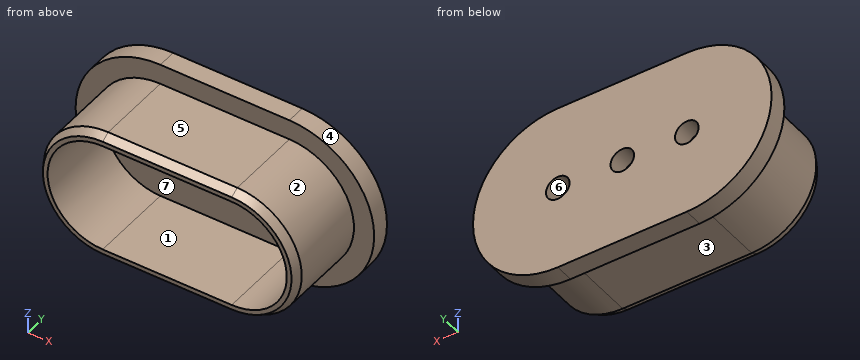
from build123d import *

# Parameters (mm, degrees)
BOSS_EXTRUDE1_DEPTH     = 4.5
SKETCH2_R               = 0.625
BOSS_EXTRUDE2_DEPTH     = 1
CHAMFER2_SIZE           = 0.25
CHAMFER2_SIZE2          = 0.433012702
SKETCH3_R               = 0.625
CUT_EXTRUDE1_DEPTH      = 1
CUT_EXTRUDE1_DEPTH_BACK = 6.5


with BuildPart() as part:
    # Sketch1 → Boss-Extrude1 (new body)
    with BuildSketch(Plane(origin=(0, 0, 0), x_dir=(1, 0, 0), z_dir=(0, 1, 0))):
        with BuildLine():
            Line((-3.425, 3.425), (3.425, 3.425))
            ThreePointArc((3.425, 3.425), (6.85, 0), (3.425, -3.425))
            Line((3.425, -3.425), (-3.425, -3.425))
            ThreePointArc((-3.425, -3.425), (-6.85, 0), (-3.425, 3.425))
        make_face()
        with BuildLine():
            Line((-3.425, 2.925), (3.425, 2.925))
            ThreePointArc((3.425, 2.925), (6.35, 0), (3.425, -2.925))
            Line((3.425, -2.925), (-3.425, -2.925))
            ThreePointArc((-3.425, -2.925), (-6.35, 0), (-3.425, 2.925))
        make_face(mode=Mode.SUBTRACT)
    extrude(amount=BOSS_EXTRUDE1_DEPTH)

    # Sketch2 → Boss-Extrude2 (add)
    with BuildSketch(Plane(origin=(0, 4.5, 0), x_dir=(1, 0, 0), z_dir=(0, 1, 0))):
        with BuildLine():
            Line((-3.425, 4.5), (3.425, 4.5))
            ThreePointArc((3.425, 4.5), (7.925, 0), (3.425, -4.5))
            Line((3.425, -4.5), (-3.425, -4.5))
            ThreePointArc((-3.425, -4.5), (-7.925, 0), (-3.425, 4.5))
        make_face()
        with Locations((-3.425, 0)):
            Circle(SKETCH2_R, mode=Mode.SUBTRACT)
        with Locations((3.425, 0)):
            Circle(SKETCH2_R, mode=Mode.SUBTRACT)
    extrude(amount=BOSS_EXTRUDE2_DEPTH)

    # Chamfer2
    chamfer2_edges = [part.edges().sort_by_distance(p)[0] for p in [
        (0, 0, 3.425),
        (-6.85, 0, 0),
        (0, 0, -3.425),
        (6.85, 0, 0),
    ]]
    chamfer2_side = [part.faces().sort_by_distance(p)[0] for p in [
        (0, 0, -3.271829344),
    ]]
    chamfer(chamfer2_edges, length=CHAMFER2_SIZE, length2=CHAMFER2_SIZE2, reference=chamfer2_side[0])

    # Sketch3 → Cut-Extrude1 (cut, two sides)
    with BuildSketch(Plane(origin=(0, 5.5, 0), x_dir=(1, 0, 0), z_dir=(0, 1, 0))) as cut_extrude1_sk:
        Circle(SKETCH3_R)
    extrude(amount=CUT_EXTRUDE1_DEPTH, mode=Mode.SUBTRACT)
    extrude(cut_extrude1_sk.sketch, amount=-CUT_EXTRUDE1_DEPTH_BACK, mode=Mode.SUBTRACT)


solid = part.part
Model file for the job. Use its own axes, mm. Face numbers are marked on the shaded views. A direction names the side the tool comes from. Give positions to 0.01 mm unless a question says otherwise; leave off trailing zeros. Write each loop counter-clockwise with the first axis right and the second up, starting at its lowest first coordinate (ties: lowest second). Pieces come first, ordered by that corner, then holes. Notation, with made-up numbers: (88.25, 87) -> (124.25, 87) arc R21 cw to (124.25, 108) -> close; hole circle Ø10 at (42.5, 48). An arc over 180 degrees is marked (long way). Write item = value, one per line.
(1) Slice it at A-A, the plane x = 0. Give the cut face in (y, z) (3 decimals).
Determined:
outline = (0, -3.175) -> (0.433, -3.425) -> (4.5, -3.425) -> (4.5, -4.5) -> (5.5, -4.5) -> (5.5, -0.625) -> (4.5, -0.625) -> (4.5, -2.925) -> (0, -2.925) -> close; (0, 2.925) -> (4.5, 2.925) -> (4.5, 0.625) -> (5.5, 0.625) -> (5.5, 4.5) -> (4.5, 4.5) -> (4.5, 3.425) -> (0.433, 3.425) -> (0, 3.175) -> close
(2) Mould opens along Z. For the marked faces 4, 5, 6 and 7 say: released by +Z, released by -Z, zero draft, split by the parting line, or undercut.
Determined:
face_4 = split by the parting line
face_5 = released by +Z
face_6 = undercut
face_7 = undercut
(3) Tool access for the marked faces 1, 2 and 3: list every direction of +Z, -Z, +X, -X, +Y, -Y with a clear straight run to the whole face (end or side of a thin tool).
Determined:
face_1 = -Y
face_2 = +X, -Y
face_3 = -Z, +X, -X, -Y
(4) Probe line 1 along X through (y, z) = (4.9, 0) (3 decimals); line 2 along Z through (x, y) = (-3.5, 3.9); line 3 along Z through (x, y) = (0, 5.25) (3 decimals). List the from-to ranges inside material, lowest first.
Determined:
line_1 = -7.925 to -4.05, -2.8 to -0.625, 0.625 to 2.8, 4.05 to 7.925
line_2 = -3.42 to -2.92, 2.92 to 3.42
line_3 = -4.5 to -0.625, 0.625 to 4.5
(5) Slice it at D-D, the plane y = 4.9. Give the cut face in (x, z) (3 decimals).
Determined:
outline = (-3.425, -4.5) -> (3.425, -4.5) arc R4.5 ccw to (3.425, 4.5) -> (-3.425, 4.5) arc R4.5 ccw to start; hole circle Ø1.25 at (-3.425, 0); hole circle Ø1.25 at (0, 0); hole circle Ø1.25 at (3.425, 0)
(6) Flat gauge pins, fed straight in: P1, Ø1.2, axis at x = 0, y = 2, coming from the -Z side (3 decimals); P2, Ø1.5, axis at x = 5, z = -1, coming from the -Y side; P3, Ø2, axis at x = 3.425, z = 0, coming from the +Y side; P4, Ø3, axis at y = 4.5, z = 2.5, coming from the +X side. Where does each tip first touch, or does it go through?
Determined:
P1 = -3.425
P2 = 4.5
P3 = 5.5
P4 = 7.81
(7) Slice it at C-C, the plane y = 3.35. Give the cut face in (x, z) (3 decimals), then the cut area to 3 significant figures.
Determined:
outline = (-3.425, -3.425) -> (3.425, -3.425) arc R3.425 ccw to (3.425, 3.425) -> (-3.425, 3.425) arc R3.425 ccw to start; hole (-3.425, -2.925) -> (3.425, -2.925) arc R2.925 ccw to (3.425, 2.925) -> (-3.425, 2.925) arc R2.925 ccw to start
area = 16.8 mm2
(8) Slice it at B-B, the plane z = 0. Give the cut face in (x, y) (3 decimals), then the cut area to 3 significant figures.
Determined:
outline = (-7.925, 4.5) -> (-6.85, 4.5) -> (-6.85, 0.433) -> (-6.6, 0) -> (-6.35, 0) -> (-6.35, 4.5) -> (-4.05, 4.5) -> (-4.05, 5.5) -> (-7.925, 5.5) -> close; (-2.8, 4.5) -> (-0.625, 4.5) -> (-0.625, 5.5) -> (-2.8, 5.5) -> close; (0.625, 4.5) -> (2.8, 4.5) -> (2.8, 5.5) -> (0.625, 5.5) -> close; (4.05, 4.5) -> (6.35, 4.5) -> (6.35, 0) -> (6.6, 0) -> (6.85, 0.433) -> (6.85, 4.5) -> (7.925, 4.5) -> (7.925, 5.5) -> (4.05, 5.5) -> close
area = 16.5 mm2
